The drawing under review shows one solid part. Ordinate dimensions are in mm from its lowest x, y, z. Coordinates: 2 decimals unless noted, no trailing zeros. Loops run counter-clockwise (first coordinate to the right, second up) from the corner with the lowest first, then second, coordinate; pieces in that order, holes last. Notation, with made-up numbers: M 54,11.25 L 76,11.25 A27 ccw 76,50.25 Z; hole C 86.5,-21 d10. An arc over 180 degrees is marked long. Put each result on its own line as item: value.
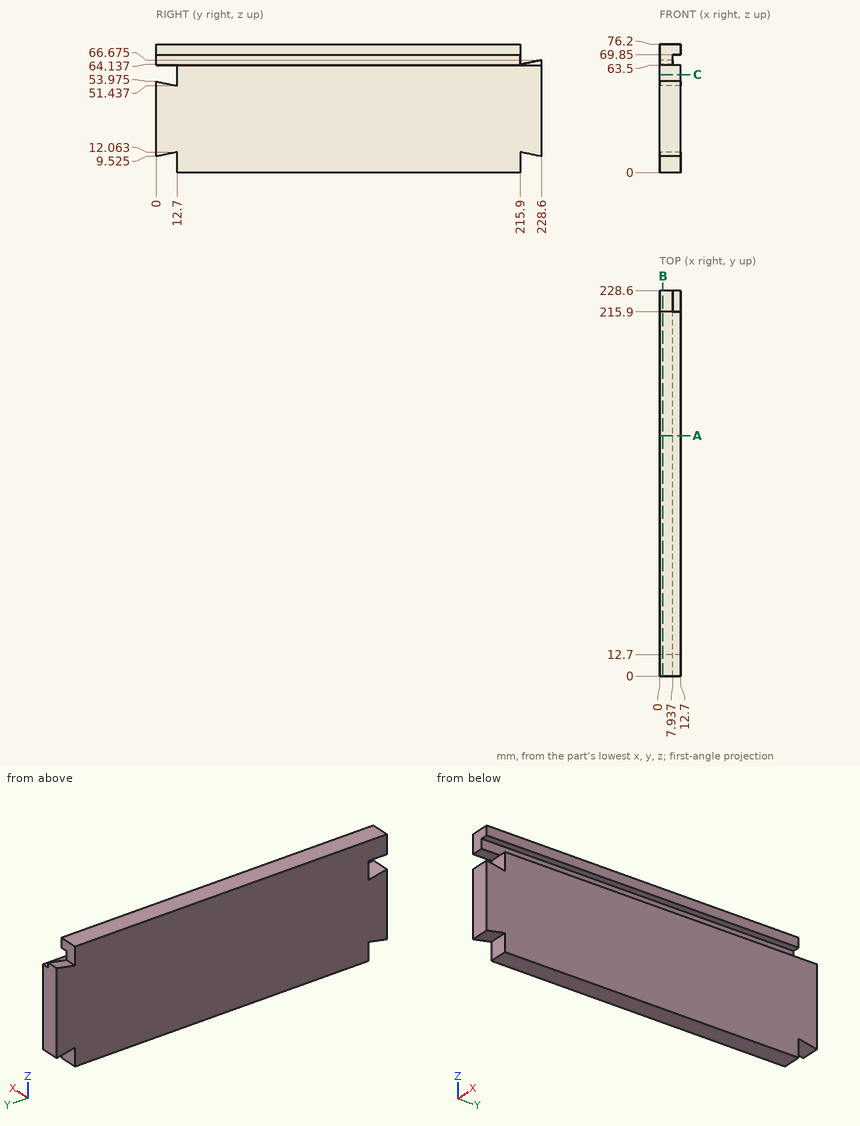
(1) Add section A-A (y = 142.5). Write out the cut boundary in (x, z).
Determined:
outline: M 0,0 L 12.7,0 L 12.7,63.5 L 7.94,63.5 L 7.94,69.85 L 12.7,69.85 L 12.7,76.2 L 0,76.2 Z
(2) For pin 1 (4 mm diameter, centred on x = 9.5, y = 74.5, fed in from -Z); pin 2 (3.5 mm diameter, centred on x = 6.5, z = 4, fed in from -Y); pin 3 (1.9 mm diameter, centred on y = 93.5, z = 66.5, fed in from +X), all flat-tipped, find the tip position at first contact; note any pin that passes through.
Determined:
pin 1: stops at z = 0
pin 2: stops at y = 12.7
pin 3: stops at x = 7.94
(3) Wall thickness on line 1 along Z through (x, y) = (12, 23.5); line 2 along Y through (x, z) = (8.25, 58); line 3 along Y through (x, z) = (6.5, 72): over which ranges is each line inside the solid? List them lowest first. Write a range as [from, to].
Determined:
line 1: z = [0, 63.5], [69.85, 76.2]
line 2: y = [12.7, 228.6]
line 3: y = [0, 215.9]
(4) Add section C-C (z = 58). Write out the cut boundary in (x, y).
Determined:
outline: M 0,12.7 L 12.7,12.7 L 12.7,228.6 L 0,228.6 Z
(5) Add section B-B (x = 2). Write out the cut boundary in (y, z) (1 decimal).
Determined:
outline: M 0,9.5 L 12.7,12.1 L 12.7,0 L 215.9,0 L 215.9,12.1 L 228.6,9.5 L 228.6,66.7 L 215.9,64.1 L 215.9,76.2 L 0,76.2 L 0,63.5 L 12.7,63.5 L 12.7,51.4 L 0,54 Z
